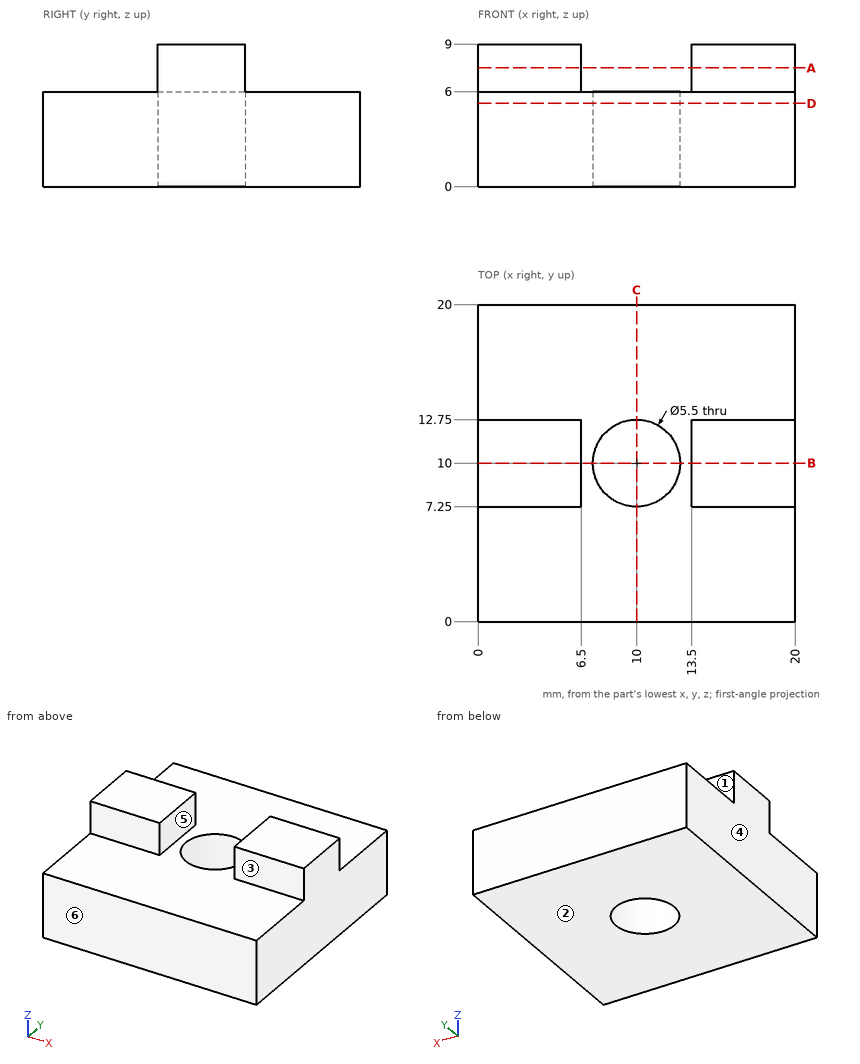
Part print with two shaded views. Sizes in mm from the minimum x, y, z corner. A direction names the side the tool comes from. Round coordinates to 2 decimals unless told otherwise and drop trailing zeros. Order: outer loops, then holes, each group sorted by start corner. A loop starts at its lowest first (then second) coordinate and runs counter-clockwise, first axis right, second up. Notation, with made-up numbers: M -25,-13.5 L -6,-13.5 A26 ccw -6,2.5 Z; hole C 49,62.25 d11. An arc over 180 degrees is marked long. Answer in a Markdown table with one row per item. Add a question column.
Q1. Mould opens along X. For the marked faces 4, 5 and 6 say: +X half, -X half, draft (parallel to the pull), parting line (faces both ways), or undercut.
Q2. Pin check, flat tips, straight feed: pin 1 (1 mm diameter, centred on x = 11.5, y = 13.5, fed in from -Z); pin 2 (0.9 mm diameter, centred on x = 2, z = 7, fed in from -Y); pin 3 (3.5 mm diameter, centred on x = 3.5, z = 8, fed in from +Y). Stop position of each tip, or through.
Q3. Wall check: L1, parallel to Y at x = 10, z = 4.05; L2, parallel to Z at x = 1.75, y = 2. Give the ranges that are in metal, low to high. Write a range as from..to.
Q4. Cut at A-A on z = 7.5. Give the cut face in (x, y), and give its area (3 significant figures).
Q5. 3-axis set-ups, long thin cutter, end or side, ignore diameter. For the marked faces 1, 2 and 3: which of +Z, -Z, +X, -X, +Y, -Y reach the whole face in a straight line?
Q6. Cut at B-B on y = 10. Give the cut face in (x, z), and give its area (3 significant figures).
Q7. Cut at D-D on z = 5.25. Give the cut face in (x, y), and give its area (3 significant figures).
Q8. Cut at C-C on x = 10. Give the cut face in (y, z), and give its area (3 significant figures).
Established:
| question | item | result |
|---|---|---|
| 1 | face 4 | -X half |
| 1 | face 5 | undercut |
| 1 | face 6 | draft |
| 2 | pin 1 | stops at z = 0 |
| 2 | pin 2 | stops at y = 7.25 |
| 2 | pin 3 | stops at y = 12.75 |
| 3 | L1 | y = 0..7.25, 12.75..20 |
| 3 | L2 | z = 0..6 |
| 4 | outline | M 0,7.25 L 6.5,7.25 L 6.5,12.75 L 0,12.75 Z; M 13.5,7.25 L 20,7.25 L 20,12.75 L 13.5,12.75 Z |
| 4 | area | 71.5 mm2 |
| 5 | face 1 | +Z, +X, -X, +Y |
| 5 | face 2 | -Z, +X, -X, +Y, -Y |
| 5 | face 3 | +Z, +X, -X, -Y |
| 6 | outline | M 0,0 L 7.25,0 L 7.25,6 L 6.5,6 L 6.5,9 L 0,9 Z; M 12.75,0 L 20,0 L 20,9 L 13.5,9 L 13.5,6 L 12.75,6 Z |
| 6 | area | 126 mm2 |
| 7 | outline | M 0,0 L 20,0 L 20,20 L 0,20 Z; hole C 10,10 d5.5 |
| 7 | area | 376 mm2 |
| 8 | outline | M 0,0 L 7.25,0 L 7.25,6 L 0,6 Z; M 12.75,0 L 20,0 L 20,6 L 12.75,6 Z |
| 8 | area | 87.0 mm2 |
